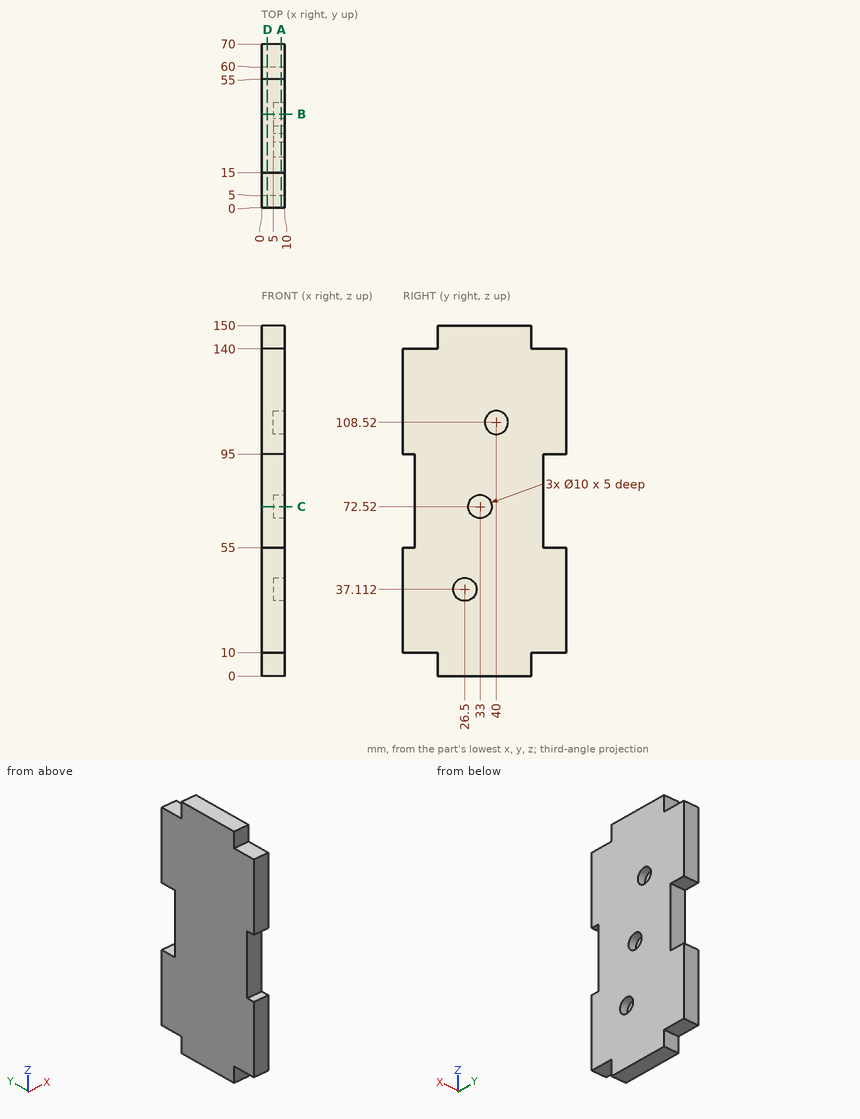
Here's the drawing with two shaded views (mm, measured from the low corner). I have some questions. Give positions to 0.01 mm unless a question says otherwise; leave off trailing zeros. Order: outer loops, then holes, each group sorted by start corner. A loop starts at its lowest first (then second) coordinate and runs counter-clockwise, first axis right, second up. Notation, with made-up numbers: (27, -13) -> (66, -13) arc R32 cw to (66, 19) -> close; hole circle Ø3 at (-7, -29.75). An arc over 180 degrees is marked (long way). One line per item, written item: value. Start each with the question number.
1. Imagine slicing it at C-C, the plane z = 72.52. List the corners of the cut face in (x, y) for me, plus the area to 3 significant figures.
2. Will these pins go through, and if not, where does the flat tip stop? pin 1 Ø5 at (x, z) = (7.5, 145) entering from +Y; pin 2 Ø6 at (y, z) = (40, 108.52) entering from +X; pin 3 Ø3 at (x, y) = (5.5, 60) entering from +Z.
3. Imagine slicing it at D-D, the plane x = 2.5. List the corners of the cut face in (y, z) for me.
4. Imagine slicing it at A-A, the plane x = 8.5. List the corners of the cut face in (y, z) for me, plus the area to 3 significant figures.
5. I need wall thicknesses on probe 1 along Y at (x, z) = (8.65, 72.52); probe 2 along Y at (x, z) = (7.5, 108.52); probe 3 along X at (y, z) = (34, 70.5). Which ranges of each line are inside material? Lowest first, please. Write a range as from..to.
6. Imagine slicing it at B-B, the plane y = 40. List the corners of the cut face in (x, z) for me.
Values follow:
1. outline: (0, 5) -> (10, 5) -> (10, 28) -> (5, 28) -> (5, 38) -> (10, 38) -> (10, 60) -> (0, 60) -> close
1. area: 500 mm2
2. pin 1: stops at y = 55
2. pin 2: stops at x = 5
2. pin 3: stops at z = 140
3. outline: (0, 10) -> (15, 10) -> (15, 0) -> (55, 0) -> (55, 10) -> (70, 10) -> (70, 55) -> (60, 55) -> (60, 95) -> (70, 95) -> (70, 140) -> (55, 140) -> (55, 150) -> (15, 150) -> (15, 140) -> (0, 140) -> (0, 95) -> (5, 95) -> (5, 55) -> (0, 55) -> close
4. outline: (0, 10) -> (15, 10) -> (15, 0) -> (55, 0) -> (55, 10) -> (70, 10) -> (70, 55) -> (60, 55) -> (60, 95) -> (70, 95) -> (70, 140) -> (55, 140) -> (55, 150) -> (15, 150) -> (15, 140) -> (0, 140) -> (0, 95) -> (5, 95) -> (5, 55) -> (0, 55) -> close; hole circle Ø10 at (26.5, 37.11); hole circle Ø10 at (33, 72.52); hole circle Ø10 at (40, 108.52)
4. area: 9,060 mm2
5. probe 1: y = 5..28, 38..60
5. probe 2: y = 0..35, 45..70
5. probe 3: x = 0..5
6. outline: (0, 0) -> (10, 0) -> (10, 103.52) -> (5, 103.52) -> (5, 113.52) -> (10, 113.52) -> (10, 150) -> (0, 150) -> close
